```python
from build123d import *

# Parameters (mm, degrees)
F0_W     = 152.4
F0_H     = 88.9
F1_DEPTH = 127
F3_DEPTH = 152.4


with BuildPart() as f1:
    # F0 (on Front) → F1 (new body)
    with BuildSketch(Plane.XZ):
        Rectangle(F0_W, F0_H)
    extrude(amount=F1_DEPTH)

    # F2 (on face) → F3 (join)
    with BuildSketch(Plane.YZ.offset(76.2)):
        Polygon((-63.5, 106.667039), (-127, 44.45), (0, 44.45), align=None)
    extrude(amount=-F3_DEPTH)


solid = f1.part
```
Can you work these out from the model? Positions are in its coordinate system, mm. Give positions to 0.01 mm unless a question says otherwise; leave off trailing zeros. Loops run counter-clockwise (first coordinate to the right, second up) from the corner with the lowest first, then second, coordinate; pieces in that order, holes last. Notation, with made-up numbers: M 21,35.25 L 44,35.25 A23 ccw 44,50.25 Z; hole C 57.25,45 d3. An arc over 180 degrees is marked long. One line per item, written item: value.
(1) Suppose I cut it at B-B on y = -106.5. List the corners of the cut face in (x, z) for me.
Returned:
outline: M -76.2,-44.45 L 76.2,-44.45 L 76.2,64.54 L -76.2,64.54 Z
(2) Suppose I cut it at C-C on z = 96.5. List the corners of the cut face in (x, y) for me.
Returned:
outline: M -76.2,-73.88 L 76.2,-73.88 L 76.2,-53.12 L -76.2,-53.12 Z
(3) Suppose I cut it at A-A on x = -65. List the corners of the cut face in (y, z) for me.
Returned:
outline: M -127,-44.45 L 0,-44.45 L 0,44.45 L -63.5,106.67 L -127,44.45 Z
(4) Will these pins go through, and if not, where does the flat tip stop? pin 1 (3 mm diameter, centred on x = -11, y = -81, fed in from +Z); pin 2 (6 mm diameter, centred on x = 56.5, y = -103.5, fed in from +Z); pin 3 (5 mm diameter, centred on x = 21.5, y = -24.5, fed in from +Z).
Returned:
pin 1: z = 90.99
pin 2: z = 70.41
pin 3: z = 70.9
(5) I need wall thicknesses on line 1 (Z direction, x = -9, y = -109); line 2 (Y direction, x = 52.5, z = 73); line 3 (Z direction, x = -5.5, y = -49.5). Which ranges of each line are inside material? Lowest first, please.
Returned:
line 1: -44.45 to 62.09
line 2: -97.86 to -29.14
line 3: -44.45 to 92.95
